from build123d import *

# Parameters (mm, degrees)
CROQUIS1_R              = 9
SALIENTE_EXTRUIR1_DEPTH = 3
CROQUIS2_R              = 3.975
SALIENTE_EXTRUIR2_DEPTH = 9
SALIENTE_EXTRUIR3_DEPTH = 42
REDONDEO1_R             = 0.8


with BuildPart() as part:
    # Croquis1 → Saliente-Extruir1 (new body)
    with BuildSketch(Plane(origin=(0, 0, 0), x_dir=(1, 0, 0), z_dir=(0, 1, 0))):
        with Locations(Location((0, 0, 0), (0, 0, 270))):
            Circle(CROQUIS1_R)
    extrude(amount=SALIENTE_EXTRUIR1_DEPTH)

    # Croquis2 → Saliente-Extruir2 (add)
    with BuildSketch(Plane(origin=(0, 3, 0), x_dir=(1, 0, 0), z_dir=(0, 1, 0))):
        with Locations(Location((0, 0, 0), (0, 0, 270))):
            Circle(CROQUIS2_R)
    extrude(amount=SALIENTE_EXTRUIR2_DEPTH)

    # Croquis3 → Saliente-Extruir3 (add)
    with BuildSketch(Plane(origin=(0, 12, 0), x_dir=(1, 0, 0), z_dir=(0, 1, 0))):
        Polygon((-2.949727384, -2.664532485), (0.832689129, -3.886805091), (3.782416513, -1.222272606), (2.949727384, 2.664532485), (-0.832689129, 3.886805091), (-3.782416513, 1.222272606), align=None)
    extrude(amount=SALIENTE_EXTRUIR3_DEPTH)

    # Redondeo1
    redondeo1_edges = [part.edges().sort_by_distance(p)[0] for p in [
        (-1.058519127, 54, 3.275668788),
        (2.307552821, 54, 2.554538849),
        (3.366071948, 54, -0.721129939),
        (1.058519127, 54, -3.275668788),
        (-2.307552821, 54, -2.554538849),
        (-3.366071948, 54, 0.721129939),
    ]]
    fillet(redondeo1_edges, radius=REDONDEO1_R)


solid = part.part
Build history of the part. All positions in model axes, mm. A direction names the side the tool comes from. Round coordinates to 2 decimals unless told otherwise and drop trailing zeros. Write each loop counter-clockwise with the first axis right and the second up, starting at its lowest first coordinate (ties: lowest second). Pieces come first, ordered by that corner, then holes. Notation, with made-up numbers: (64.5, -2) -> (106.5, -2) arc R19 cw to (106.5, 33) -> close; hole circle Ø5 at (47, 89). An arc over 180 degrees is marked (long way). Use one line per item in the form item = value.
Q1. Drill centre lines: L1, parallel to Y at x = -6.75, z = 4.75; L2, parallel to X at y = 9, z = 1.25; L3, parallel to X at y = 41.5, z = 2. Where is each one in solid material? Low to high.
Conclusion:
L1 = 0 to 3
L2 = -3.77 to 3.77
L3 = -3.09 to 2.92
Q2. Band-saw the part on C-C, the plane y = 7.5. Write the cut outline in (x, z) (3 decimals), then the cut area to 3 significant figures.
Conclusion:
outline = circle Ø7.95 at (0, 0)
area = 49.6 mm²
Q3. Tool access for faces 1 (the flat face through (-2.4, 12, -2.8)), 2 (the flat face through (1.08, 32.31, -3.27)), 3 (the flat face through (-2, 3, 4)), 4 (the flat face through (-3.6, 12, 0.7)), 5 (the flat face through (2.29, 32.31, 2.57)): list every direction of +Z, -Z, +X, -X, +Y, -Y with a clear straight run to the whole face (end or side of a thin tool).
Conclusion:
face_1 = -Z, -X, +Y
face_2 = -Z, +X, +Y
face_3 = +Y
face_4 = +Z, -X, +Y
face_5 = +Z, +X, +Y
Q4. Band-saw the part on A-A, the plane y = 46.5. Write the cut outline in (x, z), then the cut area to 3 significant figures.
Conclusion:
outline = (-3.78, -1.22) -> (-0.83, -3.89) -> (2.95, -2.66) -> (3.78, 1.22) -> (0.83, 3.89) -> (-2.95, 2.66) -> close
area = 41.1 mm²
Q5. Drop flat-ended pins along their axis: P1, Ø4, axis at y = 16, z = -5, coming from the -X side; P2, Ø4, axis at y = 43.5, z = 1.5, coming from the -X side; P3, Ø5.5, axis at x = 1.5, z = 4.5, coming from the +Y side; P4, Ø4, axis at x = -6, y = 13, coming from the -Z side. Give the stop position or say it passes through.
Conclusion:
P1 = -1.81
P2 = -3.63
P3 = 54
P4 = through
Q6. Two-plate mould, pull along Z, no slides. Class faces 6 (the flat face through (3.372, 32.312, -0.694)), 7 (the flat face through (-1.08, 32.31, 3.27)), 8 (the flat face through (0, 54, 0)): released by +Z, released by -Z, zero draft, split by the parting line, or undercut.
Conclusion:
face_6 = released by -Z
face_7 = released by +Z
face_8 = zero draft
Q7. Band-saw the part on B-B, the plane x = 5.5. Write the cut outline in (y, z), then the cut area to 3 significant figures.
Conclusion:
outline = (0, -7.12) -> (3, -7.12) -> (3, 7.12) -> (0, 7.12) -> close
area = 42.7 mm²
